```python
from build123d import *

# Parameters (mm, degrees)
SKETCH1_R           = 11.5
SKETCH1_R_2         = 1.75
SKETCH1_R_3         = 6.25
BOSS_EXTRUDE1_DEPTH = 3
SKETCH2_W           = 486
SKETCH2_H           = 70
BOSS_EXTRUDE2_DEPTH = 4
CHAMFER1_SIZE       = 10


with BuildPart() as part:
    # Sketch1 → Boss-Extrude1 (new body)
    with BuildSketch(Plane(origin=(0, 0, 0), x_dir=(1, 0, 0), z_dir=(0, 1, 0))):
        Polygon((-221.627821886, -114.515571385), (-221.627821886, 245.484428615), (-171.627821886, 245.484428615), (-171.627821886, 295.484428615), (318.372178114, 295.484428615), (318.372178114, 245.484428615), (368.372178114, 245.484428615), (368.372178114, -114.515571385), align=None)
        with Locations(Location((-106.627821886, 175.484428615, 0), (0, 0, 270))):
            Circle(SKETCH1_R, mode=Mode.SUBTRACT)
        with Locations(Location((-122.127821886, 190.984428615, 0), (0, 0, 270))):
            Circle(SKETCH1_R_2, mode=Mode.SUBTRACT)
        with Locations(Location((-91.127821886, 190.984428615, 0), (0, 0, 270))):
            Circle(SKETCH1_R_2, mode=Mode.SUBTRACT)
        with Locations(Location((-91.127821886, 159.984428615, 0), (0, 0, 270))):
            Circle(SKETCH1_R_2, mode=Mode.SUBTRACT)
        with Locations(Location((-122.127821886, 159.984428615, 0), (0, 0, 270))):
            Circle(SKETCH1_R_2, mode=Mode.SUBTRACT)
        with Locations(Location((268.872178114, 159.984428615, 0), (0, 0, 90))):
            Circle(SKETCH1_R_2, mode=Mode.SUBTRACT)
        with Locations(Location((237.872178114, 159.984428615, 0), (0, 0, 90))):
            Circle(SKETCH1_R_2, mode=Mode.SUBTRACT)
        with Locations(Location((237.872178114, 190.984428615, 0), (0, 0, 90))):
            Circle(SKETCH1_R_2, mode=Mode.SUBTRACT)
        with Locations(Location((268.872178114, 190.984428615, 0), (0, 0, 90))):
            Circle(SKETCH1_R_2, mode=Mode.SUBTRACT)
        with Locations(Location((253.372178114, 175.484428615, 0), (0, 0, 90))):
            Circle(SKETCH1_R, mode=Mode.SUBTRACT)
        with Locations(Location((-66.627821886, 275.484428615, 0), (0, 0, 270))):
            Circle(SKETCH1_R_3, mode=Mode.SUBTRACT)
        with Locations(Location((213.372178114, 275.484428615, 0), (0, 0, 270))):
            Circle(SKETCH1_R_3, mode=Mode.SUBTRACT)
    extrude(amount=BOSS_EXTRUDE1_DEPTH)

    # Sketch2 → Boss-Extrude2 (add)
    with BuildSketch(Plane(origin=(0, 58.757785693, 58.757785693), x_dir=(1, 0, 0), z_dir=(0, 0.7071067811865464, 0.7071067811865488))):
        with Locations((73.372178114, -113.853416735)):
            Rectangle(SKETCH2_W, SKETCH2_H)
    extrude(amount=-BOSS_EXTRUDE2_DEPTH)

    # Chamfer1
    chamfer1_edges = [part.edges().sort_by_distance(p)[0] for p in [
        (-169.627821886, -47.911688245, 162.598832506),
        (316.372178114, -47.911688245, 162.598832506),
    ]]
    chamfer(chamfer1_edges, length=CHAMFER1_SIZE)


solid = part.part
```
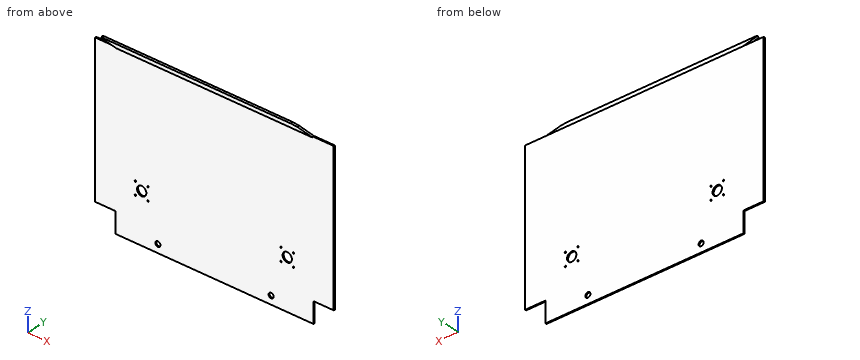
Read the model definition and answer for the solid it produces. Units are mm, in the model's axes. Coordinates: 2 decimals unless noted, no trailing zeros. Loops run counter-clockwise (first coordinate to the right, second up) from the corner with the lowest first, then second, coordinate; pieces in that order, holes last. Notation, with made-up numbers: (72.25, -35.5) - (92.25, -35.5) arc R25 ccw to (92.25, -7.5) - close; hole circle Ø6 at (6.5, 53). An arc over 180 degrees is marked (long way). Answer in a Markdown table with one row per item.
1. Find section C-C, the plane y = -10. Write down the section's boundary in (x, z).
Conclusion:
| item | result |
|---|---|
| outline | (-169.63, 121.86) - (316.37, 121.86) - (316.37, 127.52) - (-169.63, 127.52) - close |
2. Find section B-B, the plane z = -9. Write down the section's boundary in (x, y).
Conclusion:
| item | result |
|---|---|
| outline | (-221.63, 0) - (368.37, 0) - (368.37, 3) - (-221.63, 3) - close |
3. Straight lines are drawn through the part: line 1 (Y direction, x = 161, z = -125); line 2 (Z direction, x = 209, y = -39.5); line 3 (Z direction, x = 45.5, y = -33). For each, find the intervals that lie inside material, in ascending order.
Conclusion:
| item | result |
|---|---|
| line 1 | y = 0 to 3 |
| line 2 | z = 151.36 to 157.02 |
| line 3 | z = 144.86 to 150.52 |
4. Given pin 1 (5.5 mm diameter, centred on x = -91.13, z = -159.98, fed in from -Y); pin 2 (13.5 mm diameter, centred on y = -19, z = 137, fed in from -X); pin 3 (0.9 mm diameter, centred on x = -187.5, y = 1, fed in from +Z), each flat-ended and moving along its own axis, determine where each tip first touches the part or whether it passes through.
Conclusion:
| item | result |
|---|---|
| pin 1 | stops at y = 0 |
| pin 2 | stops at x = -169.63 |
| pin 3 | stops at z = 114.52 |
5. Find section A-A, the plane x = 161. Write down the section's boundary in (y, z).
Conclusion:
| item | result |
|---|---|
| outline | (-49.33, 161.18) - (0, 111.86) - (0, -295.48) - (3, -295.48) - (3, 114.52) - (-46.5, 164.01) - close |
